Part print with two shaded views. Sizes in mm from the minimum x, y, z corner. A direction names the side the tool comes from. Round coordinates to 2 decimals unless told otherwise and drop trailing zeros. Write each loop counter-clockwise with the first axis right and the second up, starting at its lowest first coordinate (ties: lowest second). Pieces come first, ordered by that corner, then holes. Notation, with made-up numbers: (-16.75, 74) -> (21.25, 74) arc R24 ccw to (21.25, 99) -> close; hole circle Ø5 at (-25.75, 59.25). An arc over 180 degrees is marked (long way). Return JSON: item names as keys, results as strings.
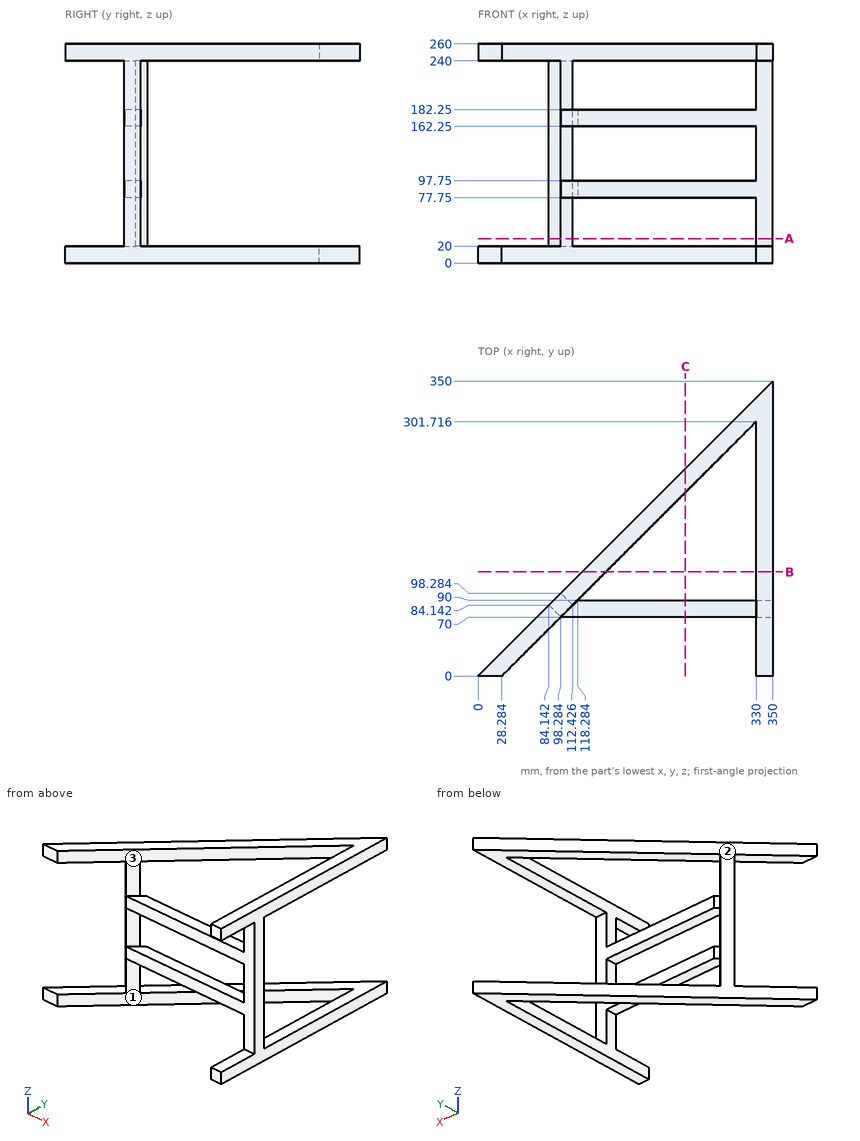
Q1. Saw through at C-C on x = 246. Count the separate pieces of the cut face and the enclosed holes in it, then the cut area to 3 significant figures.
Verdict:
{"separate pieces": "4", "enclosed holes": "0", "area": "1,930 mm²"}
Q2. Saw through at B-B on y = 123.5. List the corners of the cut face in (x, z) (1 decimal), then the cut area to 3 significant figures.
Verdict:
{"outline": "(123.5, 0) -> (151.8, 0) -> (151.8, 20) -> (123.5, 20) -> close; (123.5, 240) -> (151.8, 240) -> (151.8, 260) -> (123.5, 260) -> close; (330, 0) -> (350, 0) -> (350, 20) -> (330, 20) -> close; (330, 240) -> (350, 240) -> (350, 260) -> (330, 260) -> close", "area": "1,930 mm²"}
Q3. Saw through at A-A on z = 29. List the corners of the cut face in (x, y) (1 decimal).
Verdict:
{"outline": "(84.1, 84.1) -> (98.3, 70) -> (112.4, 84.1) -> (98.3, 98.3) -> close; (330, 70) -> (350, 70) -> (350, 90) -> (330, 90) -> close"}
Q4. 3-axis set-ups, long thin cutter, end or side, ignore diameter. For the marked faces 1, 2 and 3: which of +Z, -Z, +X, -X, +Y, -Y reach the whole face in a straight line?
Verdict:
{"face 1": "-Z, -Y", "face 2": "+Z, -Z, -X, +Y", "face 3": "+Z, -Y"}
Q5. Pin check, flat tips, straight feed: pin 1 Ø12 at (x, z) = (241, 165.5) entering from -Y; pin 2 Ø6 at (y, z) = (76.5, 144) entering from -X (1 decimal); pin 3 Ø10 at (x, y) = (339.5, 20.5) entering from -Z; pin 4 Ø16 at (x, y) = (223.5, 81.5) entering from +Z. Stop position of each tip, or through.
Verdict:
{"pin 1": "stops at y = 70", "pin 2": "stops at x = 88.8", "pin 3": "stops at z = 0", "pin 4": "stops at z = 182.25"}
Q6. Wall check: L1, parallel to Z at x = 336, y = 245.5; L2, parallel to X at y = 255, z = 11.5 (1 decimal); L3, parallel to Y at x = 336.5, z = 146.5. Give the ranges that are in metal, low to high.
Verdict:
{"L1": "z = 0 to 20, 240 to 260", "L2": "x = 255 to 283.3, 330 to 350", "L3": "y = 70 to 90"}
